Autodesk Fusion 360 part; units mm, degrees
sketch "Sketch1" plane through (0, 0, 0) normal (0, 0, 1) x (1, 0, 0)
  circle A0 centre (22, 0) radius 3.3
  line L0 (2.38, 11.6596) -> (23.5, 7.3485)
  line L1 (36, 0) -> (-21.665, 0) construction
  line L2 (2.38, -11.6596) -> (23.5, -7.3485)
  arc A1 (23.5, -7.3485) -> (23.5, 7.3485) centre (22, 0) ccw
  arc A2 (2.38, 11.6596) -> (2.38, -11.6596) centre (0, 0) ccw
  circle A3 centre (0, 0) radius 8.93
  dimension "d1" = 23.8
  dimension "d2" = 15
  dimension "d3" = 22
  dimension "d4" = 6.6
  dimension "d5" = 17.86
extrude "Extrude1" add sketch "Sketch1" along normal blind 5
extrude "Extrude2" add sketch "Sketch1" along normal blind 36.75 contours A3
equation "d8 = 5 mm + 31.75 mm"
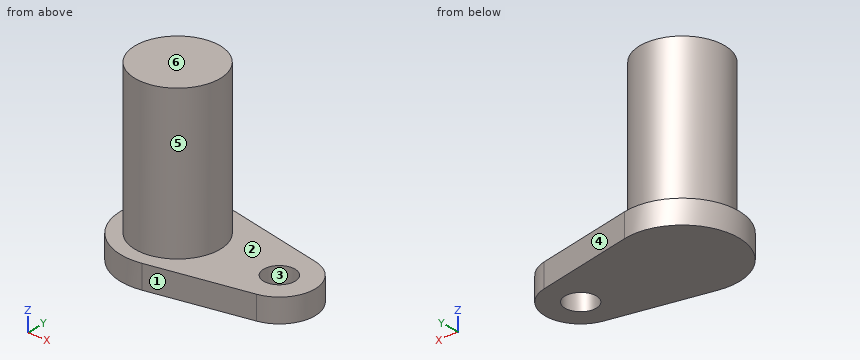
Check sheet for the modelled part. Datum: model origin and axes. Units: mm. Face numbers are marked on the shaded views. A direction names the side the tool comes from. Give positions to 0.01 mm unless a question says otherwise; leave off trailing zeros. Write each loop counter-clockwise with the first axis right and the second up, starting at its lowest first coordinate (ties: lowest second). Pieces come first, ordered by that corner, then holes. Notation, with made-up numbers: (78.25, 3.25) -> (82.25, 3.25) arc R18 ccw to (82.25, 10.25) -> close; hole circle Ø9 at (-3, 36). An arc over 180 degrees is marked (long way). Write item = value, one per line.
Item 1: Sectioned sample at D-D on x = 0. Record the boundary of the cut face in (y, z), and give its area (3 significant figures).
Output:
outline = (-11.9, 0) -> (11.9, 0) -> (11.9, 5) -> (8.93, 5) -> (8.93, 36.75) -> (-8.93, 36.75) -> (-8.93, 5) -> (-11.9, 5) -> close
area = 686 mm^2
Item 2: Sectioned sample at A-A on y = -1. Record the boundary of the cut face in (x, z), and give its area (3 significant figures).
Output:
outline = (-11.86, 0) -> (18.86, 0) -> (18.86, 5) -> (8.87, 5) -> (8.87, 36.75) -> (-8.87, 36.75) -> (-8.87, 5) -> (-11.86, 5) -> close; (25.14, 0) -> (29.43, 0) -> (29.43, 5) -> (25.14, 5) -> close
area = 738 mm^2
Item 3: Tool access check on the marked faces 5 and 6. Record the directions out of +Z, -Z, +X, -X, +Y, -Y that give a thin tool (end or side, any length) a straight path to the whole face; none if there is none.
Output:
face_5 = +Z
face_6 = +Z, +X, -X, +Y, -Y
Item 4: Release check for a two-part mould opening along Y. For the marked faces 1, 2, 3 and 4 record: +Y half, -Y half, draft (parallel to the pull), parting line (faces both ways), or undercut.
Output:
face_1 = -Y half
face_2 = draft
face_3 = undercut
face_4 = +Y half
Item 5: Sectioned sample at B-B on x = 22. Record the boundary of the cut face in (y, z), and give its area (3 significant figures).
Output:
outline = (-7.65, 0) -> (-3.3, 0) -> (-3.3, 5) -> (-7.65, 5) -> close; (3.3, 0) -> (7.65, 0) -> (7.65, 5) -> (3.3, 5) -> close
area = 43.5 mm^2
Item 6: Scan lines: probe 1 along Z at (x, y) = (16, -8.5); probe 2 along Y at (x, z) = (24, 4); probe 3 along Y at (x, z) = (22, 3.95). Record each from-to range of solid material in increasing order. Write a range as from..to.
Output:
probe_1 = 0..5
probe_2 = -7.23..-2.62, 2.62..7.23
probe_3 = -7.65..-3.3, 3.3..7.65
Item 7: Sectioned sample at C-C on z = 3.5. Record the boundary of the cut face in (x, y).
Output:
outline = (2.38, -11.66) -> (23.5, -7.35) arc R7.5 ccw to (23.5, 7.35) -> (2.38, 11.66) arc R11.9 ccw (long way) to start; hole circle Ø6.6 at (22, 0)
Item 8: Gauge pin test, flat ends, axial feed: pin 1 (3 mm diameter, centred on x = 0.5, z = 21, fed in from +Y); pin 2 (2 mm diameter, centred on y = 0.5, z = 12, fed in from -X); pin 3 (7.5 mm diameter, centred on x = 22, y = 0, fed in from +Z); pin 4 (12 mm diameter, centred on x = 19.5, z = 16.5, fed in from +Y). Record the tip position at first contact, or that the pin passes through.
Output:
pin_1 = 8.93
pin_2 = -8.93
pin_3 = 5
pin_4 = through
